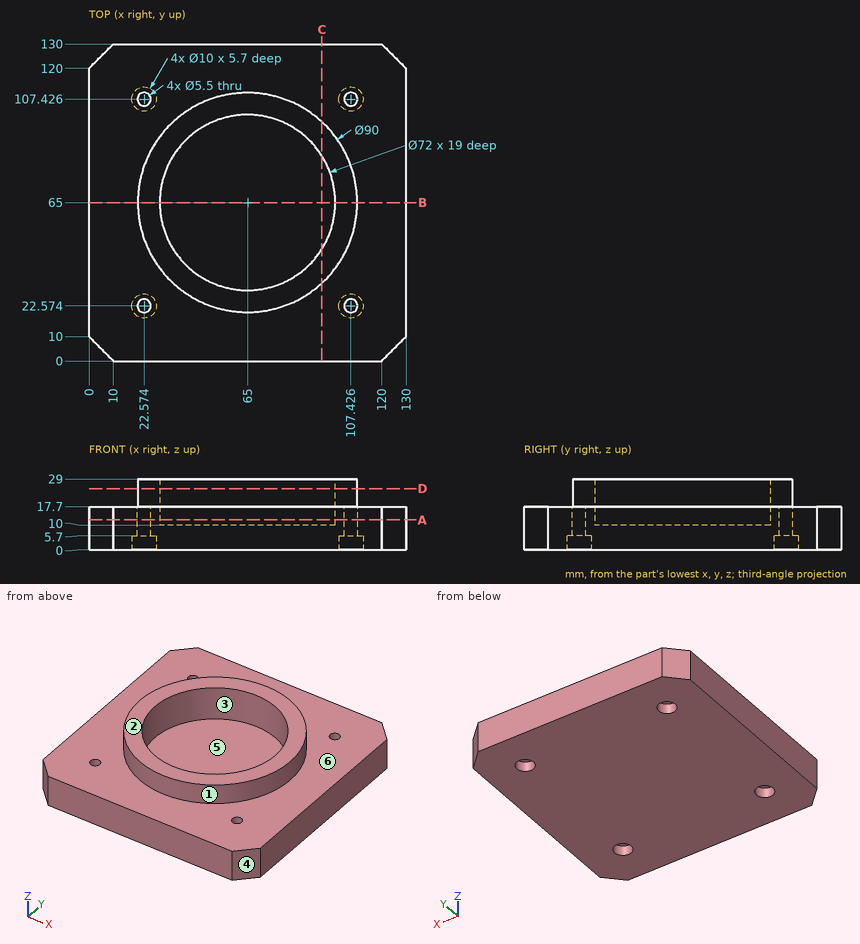
Can you work these out from the drawing? Everything is in mm from the part's minimum corner. A direction names the side the tool comes from. Coordinates: 2 decimals unless noted, no trailing zeros. Loops run counter-clockwise (first coordinate to the right, second up) from the corner with the lowest first, then second, coordinate; pieces in that order, holes last.
1) Imagine slicing it at D-D on z = 25. List the corners of the cut face in (x, y) for me, plus the area to 3 significant figures.
2) Which directions (+Z, -Z, +X, -X, +Y, -Y) give clear straight access to the entire face, cutting with the end or side of a thin tool? Please do the marked faces 1 and 2.
3) For pin 1 (3.5 mm diameter, centred on x = 107.43, y = 107.43, fed in from +Z); pin 2 (5 mm diameter, centred on x = 109, y = 21, fed in from -Z); pin 3 (1 mm diameter, centred on y = 95.5, z = 19.5, fed in from +X); pin 4 (3 mm diameter, centred on y = 27.5, z = 26, fed in from +X), each with a flat end and sliding along its axis, tell me the tip position at first contact or that it passes through.
4) Imagine slicing it at A-A on z = 12.25. List the corners of the cut face in (x, y) for me.
5) Imagine slicing it at B-B on y = 65. List the corners of the cut face in (x, z) for me, plus the area to 3 significant figures.
6) I need wall thicknesses on probe 1 along Y at (x, z) = (23, 17.25); probe 2 along Y at (x, z) = (65, 21.25); probe 3 along Z at (x, y) = (107, 110.5). Which ranges of each line are inside material? Lowest first, please.
7) Imagine slicing it at C-C on x = 95.5. List the corners of the cut face in (y, z) for me (1 decimal), plus the area to 3 significant figures.
8) Thinking about a two-plate mould opening in X: for the marked faces 3, 4, 5 and 6, which applies, pulls with the +X half, pulls with the -X half, needs draft (parallel to the pull), parting line crosses it, or undercut?
Completed:
1. outline: circle Ø90 at (65, 65); hole circle Ø72 at (65, 65)
1. area: 2,290 mm2
2. face 1: +Z
2. face 2: +Z, +X, -X, +Y, -Y
3. pin 1: passes through
3. pin 2: stops at z = 5.7
3. pin 3: stops at x = 98.54
3. pin 4: stops at x = 92
4. outline: (0, 10) - (10, 0) - (120, 0) - (130, 10) - (130, 120) - (120, 130) - (10, 130) - (0, 120) - close; hole circle Ø5.5 at (22.57, 22.57); hole circle Ø5.5 at (22.57, 107.43); hole circle Ø72 at (65, 65); hole circle Ø5.5 at (107.43, 22.57); hole circle Ø5.5 at (107.43, 107.43)
5. outline: (0, 0) - (130, 0) - (130, 17.7) - (110, 17.7) - (110, 29) - (101, 29) - (101, 10) - (29, 10) - (29, 29) - (20, 29) - (20, 17.7) - (0, 17.7) - close
5. area: 1,950 mm2
6. probe 1: y = 0 to 19.86, 25.29 to 104.71, 110.14 to 130
6. probe 2: y = 20 to 29, 101 to 110
6. probe 3: z = 5.7 to 17.7
7. outline: (0, 0) - (130, 0) - (130, 17.7) - (98.1, 17.7) - (98.1, 29) - (84.1, 29) - (84.1, 10) - (45.9, 10) - (45.9, 29) - (31.9, 29) - (31.9, 17.7) - (0, 17.7) - close
7. area: 2,320 mm2
8. face 3: undercut
8. face 4: pulls with the +X half
8. face 5: undercut
8. face 6: needs draft
